The model under review builds one solid part; all positions refer to its coordinate system, in mm. A direction names the side the tool comes from. Round coordinates to 2 decimals unless told otherwise and drop trailing zeros. Order: outer loops, then holes, each group sorted by start corner. A loop starts at its lowest first (then second) coordinate and runs counter-clockwise, first axis right, second up. Notation, with made-up numbers: M -30.75,28.25 L 21.25,28.25 A5 cw 21.25,34.25 Z; hole C -33,-13.5 d5. An arc over 180 degrees is marked long. Answer as a JSON object with one key per item and string values. Group by question number.
1) Consider section B-B, the plane x = 18.5. Write out the cut boundary in (y, z), then the cut area to 3 significant figures.
2) Consider section A-A, the plane z = 0. Write out the cut boundary in (x, y).
3) For faces 4 (the cylindrical face through (-10.49, 0.46, 162.15)), 5 (the flat face through (30, 25, 7)), 6 (the cylindrical face through (123.2, 3.2, 279.5)), 7 (the cylindrical face through (0.42, 7.509, -23.846)), list the 3-axis set-ups (+Z, -Z, +X, -X, +Y, -Y) from which the entire face can be reached by the end or side of a thin tool; tool diameter is ignored.
4) To check wall thickness, follow line 1 (Y direction, x = 0, z = 186.5); line 2 (Y direction, x = 3.5, z = 0); line 3 (Z direction, x = 178, y = 0). State the ranges of each line that lie inside material, in increasing order.
5) Insertion check: pin 1 Ø8.5 at (y, z) = (1, 294) entering from -X; pin 2 Ø2 at (y, z) = (-9.5, 243) entering from -X; pin 3 Ø12 at (y, z) = (2.5, 166.5) entering from +X. Each pin has a flat end and moves straight along its axis. Give the tip position at first contact, or say it passes through.
6) Consider section D-D, the plane x = 83.5. Write out the cut boundary in (y, z).
7) The part is to be moulded in two halves that separate along Y. For faces 1 (the cylindrical face through (0.42, -11.49, -27.712)), 2 (the cylindrical face through (3, 0, 297)), 3 (the flat face through (250, 2, 297)), say which applies: +Y half, -Y half, draft (parallel to the pull), parting line (faces both ways), or undercut.
```python
from build123d import *

# Parameters (mm, degrees)
SKETCH_1_R          = 10.5
EXTRUDE_1_DEPTH     = 300
SKETCH_2_R          = 7.5
CUT_EXTRUDE_1_DEPTH = 301
SKETCH_4_R          = 30
EXTRUDE_2_DEPTH     = 30
SKETCH_5_R          = 25
CUT_EXTRUDE_2_DEPTH = 61.0000001
SKETCH_7_R          = 10.5
SKETCH_7_R_2        = 7.5
EXTRUDE_4_DEPTH     = 250


with BuildPart() as part:
    # Эскиз1 → Бобышка-Вытянуть1 (new body)
    with BuildSketch(Plane.XY):
        Circle(SKETCH_1_R)
    extrude(amount=EXTRUDE_1_DEPTH)

    # Эскиз2 → Вырез-Вытянуть1 (cut, through all)
    with BuildSketch(Plane(origin=(0, 0, 0), x_dir=(-1, 0, 0), z_dir=(0, 0, -1))):
        Circle(SKETCH_2_R)
    extrude(amount=-CUT_EXTRUDE_1_DEPTH, mode=Mode.SUBTRACT)

    # Эскиз4 → Бобышка-Вытянуть2 (add, symmetric)
    with BuildSketch(Plane(origin=(0, 0, 0), x_dir=(0, 0, -1), z_dir=(1, 0, 0))):
        Circle(SKETCH_4_R)
    extrude(amount=EXTRUDE_2_DEPTH, both=True)

    # Эскиз5 → Вырез-Вытянуть2 (cut, through all)
    with BuildSketch(Plane(origin=(30, 0, 0), x_dir=(0, 0, -1), z_dir=(1, 0, 0))):
        Circle(SKETCH_5_R)
    extrude(amount=-CUT_EXTRUDE_2_DEPTH, mode=Mode.SUBTRACT)

    # Эскиз7 → Бобышка-Вытянуть4 (add)
    with BuildSketch(Plane(origin=(0, 0, 0), x_dir=(0, 0, -1), z_dir=(1, 0, 0))):
        with Locations((-289.5, 0)):
            Circle(SKETCH_7_R)
        with Locations((-289.5, 0)):
            Circle(SKETCH_7_R_2, mode=Mode.SUBTRACT)
    extrude(amount=EXTRUDE_4_DEPTH)


solid = part.part
```
Results list:
{
 "1": {"outline": "C 0,0 d60; C 0,289.5 d21; hole C 0,0 d50; hole C 0,289.5 d15", "area": "1,030 mm^2"},
 "2": {"outline": "M -30,-30 L 30,-30 L 30,-25 L -30,-25 Z; M -30,25 L 30,25 L 30,30 L -30,30 Z"},
 "3": {"face 4": "none", "face 5": "-Z, +X, +Y, -Y", "face 6": "+X", "face 7": "+X, -X"},
 "4": {"line 1": "-10.5 to -7.5, 7.5 to 10.5", "line 2": "-30 to -25, 25 to 30", "line 3": "279 to 282, 297 to 300"},
 "5": {"pin 1": "x = -10.5", "pin 2": "x = -6.16", "pin 3": "x = 10.5"},
 "6": {"outline": "C 0,289.5 d21; hole C 0,289.5 d15"},
 "7": {"face 1": "parting line", "face 2": "undercut", "face 3": "draft"}
}
